Answer from the drawing. Dimensions are ordinates in mm from the lowest x, y and z of the part. Coordinates: 2 decimals unless noted, no trailing zeros. Loops run counter-clockwise (first coordinate to the right, second up) from the corner with the lowest first, then second, coordinate; pieces in that order, holes last. Notation, with made-up numbers: M 57,-12 L 108,-12 A31 cw 108,26 Z; hole C 60,50 d6. An arc over 180 degrees is marked long. Answer as CSV lines item,"result". Start each with the question number.
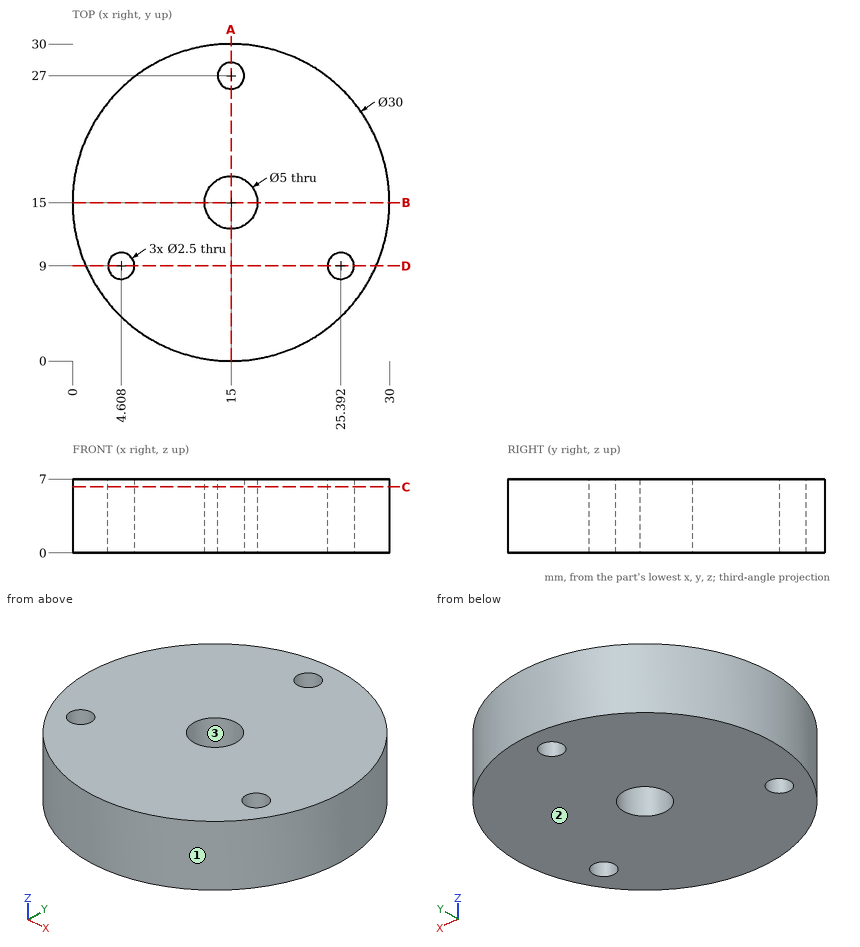
Item 1: Consider line 1 (Y direction, x = 15, z = 1.5); line 2 (Y direction, x = 17, z = 2) (1 decimal); line 3 (Y direction, x = 24.25, z = 1) (1 decimal). Determine where each line is inside the solid, lowest interval first.
Item 2: Section D-D on y = 9 is taken. Determine the outline of the cut face in (x, z).
Item 3: Section A-A on x = 15 is taken. Determine the outline of the cut face in (y, z).
Item 4: Section B-B on y = 15 is taken. Determine the outline of the cut face in (x, z), then the cut area to 3 significant figures.
Item 5: Section C-C on z = 6.25 is taken. Determine the outline of the cut face in (x, y).
Item 6: For a pull along Y with two mould halves and no side action, classify the marked faces 1, 2 and 3 as pulls with the +Y half, pulls with the -Y half, needs draft (parallel to the pull), parting line crosses it, or undercut.
Item 7: Each of these flat-tipped pins is pushed along its axis until it touches: P1, Ø1.5, axis at x = 6.5, z = 4.5, coming from the -Y side; P2, Ø1, axis at y = 24.5, z = 3.5, coming from the -X side; P3, Ø1.5, axis at x = 25.39, y = 9, coming from the -Z side; P4, Ø2, axis at y = 24.5, z = 3, coming from the -X side. Where does it stop, or does it pass through?
Results are:
1,line 1,"0 to 12.5, 17.5 to 25.75, 28.25 to 30"
1,line 2,"0.1 to 13.5, 16.5 to 29.9"
1,line 3,"3.2 to 8.5, 9.5 to 26.8"
2,outline,"M 1.25,0 L 3.36,0 L 3.36,7 L 1.25,7 Z; M 5.86,0 L 24.14,0 L 24.14,7 L 5.86,7 Z; M 26.64,0 L 28.75,0 L 28.75,7 L 26.64,7 Z"
3,outline,"M 0,0 L 12.5,0 L 12.5,7 L 0,7 Z; M 17.5,0 L 25.75,0 L 25.75,7 L 17.5,7 Z; M 28.25,0 L 30,0 L 30,7 L 28.25,7 Z"
4,outline,"M 0,0 L 12.5,0 L 12.5,7 L 0,7 Z; M 17.5,0 L 30,0 L 30,7 L 17.5,7 Z"
4,area,"175 mm²"
5,outline,"C 15,15 d30; hole C 4.61,9 d2.5; hole C 15,15 d5; hole C 15,27 d2.5; hole C 25.39,9 d2.5"
6,face 1,"parting line crosses it"
6,face 2,"needs draft"
6,face 3,"undercut"
7,P1,"y = 2.16"
7,P2,"x = 3"
7,P3,"through"
7,P4,"x = 2.64"
